from build123d import *

# Parameters (mm, degrees)
F0_W      = 165.1
F0_H      = 254
F1_DEPTH  = 63.5
F2_T      = 5.08
F0_W_2    = 25.4
F3_DEPTH  = 5.08
F5_D      = 6.35
F7_D      = 19.05
F8_W      = 182.88
F8_H      = 8.2663088166
F9_DEPTH  = 25.4
F10_W     = 182.88
F10_H     = 7.62
F11_DEPTH = 25.4


with BuildPart() as f1:
    # F0 (on Top) → F1 (new body)
    with BuildSketch(Plane.XY):
        with Locations((1.211356771, 1.3005096912)):
            Rectangle(F0_W, F0_H)
    extrude(amount=-F1_DEPTH)

    # F2
    f2_openings = [f1.faces().sort_by_distance(p)[0] for p in [
        (1.211357, -125.69949, -31.75),
        (1.211357, 1.30051, 0),
    ]]
    offset(amount=F2_T, openings=f2_openings, kind=Kind.INTERSECTION)

    # F0 (on Top) → F3 (join)
    with BuildSketch(Plane.XY):
        with Locations((-94.038643229, 1.3005096912)):
            Rectangle(F0_W_2, F0_H)
        Polygon((-106.738643229, 128.3005096912), (-81.338643229, 128.3005096912), (83.761356771, 128.3005096912), (109.161356771, 128.3005096912), (109.161356771, 153.7005096912), (-106.738643229, 153.7005096912), align=None)
        with Locations((96.461356771, 1.3005096912)):
            Rectangle(F0_W_2, F0_H)
    extrude(amount=F3_DEPTH)

    # F5 (through all)
    with Locations(Plane(origin=(0, 0, 0), x_dir=(1, 0, 0), z_dir=(0, 0, -1))):
        with Locations((-94.038643229, -64.8005096912), (-94.038643229, 62.1994903088), (-55.938643229, -141.0005096912), (96.461356771, 62.1994903088), (96.461356771, -64.8005096912), (58.361356771, -141.0005096912)):
            Hole(F5_D / 2)

    # F7 (through all)
    with Locations(Plane.XY.offset(-63.5)):
        with Locations((-41.275, 106.0755096912), (41.275, 106.0755096912), (41.275, 67.9755096912), (0, 87.0255096912), (-41.275, 67.9755096912), (0, 48.9255096912), (41.275, 29.8755096912), (-41.275, 29.8755096912), (0, 10.8255096912), (-41.275, -8.2244903088), (41.275, -8.2244903088), (0, -27.2744903088), (41.275, -46.3244903088), (-41.275, -46.3244903088), (0, -65.3744903088), (41.275, -84.4244903088), (-41.275, -84.4244903088)):
            Hole(F7_D / 2)

    # F8 (on face) → F9 (cut)
    with BuildSketch(Plane(origin=(-86.418643229, 0, 0), x_dir=(0, -1, 0), z_dir=(-1, 0, 0))):
        with Locations((-3.8405096912, -18.1031544083)):
            Rectangle(F8_W, F8_H)
        with Locations((-3.8405096912, -33.9944171529)):
            Rectangle(F8_W, F8_H)
        with Locations((-3.8405096912, -49.8807259695)):
            Rectangle(F8_W, F8_H)
    extrude(amount=-F9_DEPTH, mode=Mode.SUBTRACT)

    # F10 (on face) → F11 (cut)
    with BuildSketch(Plane.YZ.offset(88.841356771)):
        with Locations((3.8405096912, -19.7358)):
            Rectangle(F10_W, F10_H)
        with Locations((3.8405096912, -34.9758)):
            Rectangle(F10_W, F10_H)
        with Locations((3.8405096912, -50.2158)):
            Rectangle(F10_W, F10_H)
    extrude(amount=-F11_DEPTH, mode=Mode.SUBTRACT)


solid = f1.part
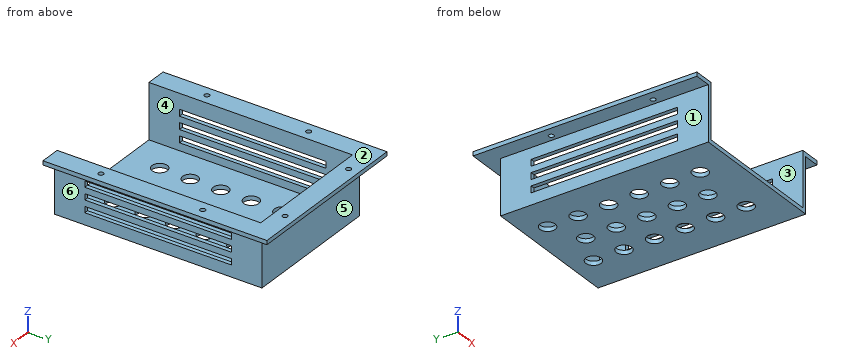
Design review of the part built by this model. Coordinates are the model's own, in mm. Face numbers are marked on the shaded views. A direction names the side the tool comes from. Round coordinates to 2 decimals unless told otherwise and drop trailing zeros. Loops run counter-clockwise (first coordinate to the right, second up) from the corner with the lowest first, then second, coordinate; pieces in that order, holes last. Notation, with made-up numbers: (47, 39) -> (51, 39) arc R16 cw to (51, 47) -> close; hole circle Ø4 at (-17, 79). An arc over 180 degrees is marked (long way). Use one line per item in the form item = value. Start each with the question number.
Q1. Wall thickness on line 1 along Y through (x, z) = (0, -65.5); line 2 along Y through (x, z) = (88, -33); line 3 along X through (y, z) = (73, -2.5): over which ranges is each line inside the solid? List them lowest first. Write a range as [from, to].
Q2. We need section D-D on x = -66. Give the boundary of the cut face in (y, z).
Q3. We need section B-B on x = 0. Give the boundary of the cut face in (y, z), then the cut area to 3 significant figures.
Q4. We need section A-A on z = -35. Give the boundary of the cut face in (x, y).
Q5. Machinability: for the marked faces 1, 2 and 3, which of the approach directions +Z, -Z, +X, -X, +Y, -Y give a long, thin tool a straight path to every point of the face, cutting with its end or side? Answer none if there is none.
Q6. For pin 1 Ø5.5 at (x, z) = (-84.5, -48) entering from +Y; pin 2 Ø3 at (y, z) = (18, -7.5) entering from +X; pin 3 Ø2 at (x, z) = (64.5, -11) entering from -Y; pin 4 Ø25 at (x, y) = (-41.28, -84.42) entering from -Z, all flat-tipped, find the tip position at first contact; note any pin that passes through.
Q7. We need section C-C on y = 120.5. Give the boundary of the cut face in (x, z), then the cut area to 3 significant figures.
Q8. Draft analysis for pull direction X (two halves, no side actions). For the marked faces 4, 5 and 6, state which applies: +X half, -X half, draft (parallel to the pull), parting line (faces both ways), or undercut.
Calculated:
q1.line_1 = [-125.7, -74.9], [-55.85, -36.8], [-17.75, 1.3], [20.35, 39.4], [58.45, 77.5], [96.55, 133.38]
q1.line_2 = [-125.7, -87.6], [95.28, 133.38]
q1.line_3 = [-86.42, -81.34], [83.76, 88.84]
q2.outline = (-125.7, -68.58) -> (133.38, -68.58) -> (133.38, 0) -> (153.7, 0) -> (153.7, 5.08) -> (128.3, 5.08) -> (128.3, -63.5) -> (-125.7, -63.5) -> close
q3.outline = (-125.7, -68.58) -> (-74.9, -68.58) -> (-74.9, -63.5) -> (-125.7, -63.5) -> close; (-55.85, -68.58) -> (-36.8, -68.58) -> (-36.8, -63.5) -> (-55.85, -63.5) -> close; (-17.75, -68.58) -> (1.3, -68.58) -> (1.3, -63.5) -> (-17.75, -63.5) -> close; (20.35, -68.58) -> (39.4, -68.58) -> (39.4, -63.5) -> (20.35, -63.5) -> close; (58.45, -68.58) -> (77.5, -68.58) -> (77.5, -63.5) -> (58.45, -63.5) -> close; (96.55, -68.58) -> (133.38, -68.58) -> (133.38, 0) -> (153.7, 0) -> (153.7, 5.08) -> (128.3, 5.08) -> (128.3, -63.5) -> (96.55, -63.5) -> close
q3.area = 1,280 mm²
q4.outline = (-86.42, -125.7) -> (-81.34, -125.7) -> (-81.34, -87.6) -> (-86.42, -87.6) -> close; (-86.42, 95.28) -> (-81.34, 95.28) -> (-81.34, 128.3) -> (83.76, 128.3) -> (83.76, 95.28) -> (88.84, 95.28) -> (88.84, 133.38) -> (-86.42, 133.38) -> close; (83.76, -125.7) -> (88.84, -125.7) -> (88.84, -87.6) -> (83.76, -87.6) -> close
q5.face_1 = -Z, -X, +Y, -Y
q5.face_2 = +Z, +X, -X, +Y, -Y
q5.face_3 = +Z, -Y
q6.pin_1 = 133.38
q6.pin_2 = 88.84
q6.pin_3 = 128.3
q6.pin_4 = -68.58
q7.outline = (-106.74, 0) -> (-86.42, 0) -> (-86.42, -68.58) -> (88.84, -68.58) -> (88.84, 0) -> (109.16, 0) -> (109.16, 5.08) -> (83.76, 5.08) -> (83.76, -63.5) -> (-81.34, -63.5) -> (-81.34, 5.08) -> (-106.74, 5.08) -> close
q7.area = 1,790 mm²
q8.face_4 = undercut
q8.face_5 = draft
q8.face_6 = +X half
